Design review of the part built by this model. Coordinates are the model's own, in mm. Coordinates: 2 decimals unless noted, no trailing zeros. Loops run counter-clockwise (first coordinate to the right, second up) from the corner with the lowest first, then second, coordinate; pieces in that order, holes last. Notation, with made-up numbers: (6, 13) -> (32, 13) arc R7 cw to (32, 24) -> close; hole circle Ø5 at (-12, 32.25). An arc over 180 degrees is marked (long way). Use CSV: the item, a comma, the result in double quotes.
```python
from build123d import *

# Parameters (mm, degrees)
SKETCH1_R           = 1.6
SKETCH1_R_2         = 1.65
SKETCH1_R_3         = 1.5
BOSS_EXTRUDE1_DEPTH = 4
FILLET1_R           = 4
FILLET2_R           = 10


with BuildPart() as part:
    # Sketch1 → Boss-Extrude1 (new body)
    with BuildSketch(Plane.XY):
        with BuildLine():
            Line((0, 0), (96, 0))
            Line((96, 0), (96, 20))
            Line((96, 20), (80, 31.52))
            Line((80, 31.52), (80, 126))
            Line((80, 126), (16, 126))
            Line((16, 126), (16, 70.5))
            Line((16, 70.5), (36.610950109, 67.962533624))
            ThreePointArc((36.610950109, 67.962533624), (41, 63), (36.610950109, 58.037466376))
            Line((36.610950109, 58.037466376), (16, 55.5))
            Line((16, 55.5), (16, 31.52))
            Line((16, 31.52), (0, 20))
            Line((0, 20), (0, 0))
        make_face()
        with Locations((4.15, 5)):
            Circle(SKETCH1_R, mode=Mode.SUBTRACT)
        with Locations((12.65, 5)):
            Circle(SKETCH1_R, mode=Mode.SUBTRACT)
        with Locations((12.65, 15)):
            Circle(SKETCH1_R, mode=Mode.SUBTRACT)
        with Locations((4.15, 15)):
            Circle(SKETCH1_R, mode=Mode.SUBTRACT)
        with Locations(Location((91.85, 5, 0), (0, 0, 180))):
            Circle(SKETCH1_R, mode=Mode.SUBTRACT)
        with Locations(Location((83.35, 5, 0), (0, 0, 180))):
            Circle(SKETCH1_R, mode=Mode.SUBTRACT)
        with Locations(Location((83.35, 15, 0), (0, 0, 180))):
            Circle(SKETCH1_R, mode=Mode.SUBTRACT)
        with Locations(Location((91.85, 15, 0), (0, 0, 180))):
            Circle(SKETCH1_R, mode=Mode.SUBTRACT)
        with Locations((48, 3)):
            Circle(SKETCH1_R, mode=Mode.SUBTRACT)
        with Locations((23.5, 123)):
            Circle(SKETCH1_R, mode=Mode.SUBTRACT)
        with Locations((72.5, 123)):
            Circle(SKETCH1_R, mode=Mode.SUBTRACT)
        with Locations((64, 71)):
            Circle(SKETCH1_R_2, mode=Mode.SUBTRACT)
        with Locations((64, 55)):
            Circle(SKETCH1_R_2, mode=Mode.SUBTRACT)
        with Locations((46, 63)):
            Circle(SKETCH1_R_3, mode=Mode.SUBTRACT)
        with BuildLine():
            Line((45.35, 122.6), (45.35, 109.4))
            ThreePointArc((45.35, 109.4), (43.75, 107.8), (42.15, 109.4))
            Line((42.15, 109.4), (42.15, 122.6))
            ThreePointArc((42.15, 122.6), (43.75, 124.2), (45.35, 122.6))
        make_face(mode=Mode.SUBTRACT)
        with BuildLine():
            Line((50.65, 109.4), (50.65, 122.6))
            ThreePointArc((50.65, 122.6), (52.25, 124.2), (53.85, 122.6))
            Line((53.85, 122.6), (53.85, 109.4))
            ThreePointArc((53.85, 109.4), (52.25, 107.8), (50.65, 109.4))
        make_face(mode=Mode.SUBTRACT)
    extrude(amount=BOSS_EXTRUDE1_DEPTH)

    # Fillet1
    fillet1_edges = [part.edges().sort_by_distance(p)[0] for p in [
        (16, 55.5, 2),
        (16, 70.5, 2),
        (16, 126, 2),
        (80, 126, 2),
        (96, 0, 2),
        (0, 0, 2),
    ]]
    fillet(fillet1_edges, radius=FILLET1_R)

    # Fillet2
    fillet2_edges = [part.edges().sort_by_distance(p)[0] for p in [
        (0, 20, 2),
        (16, 31.52, 2),
        (80, 31.52, 2),
        (96, 20, 2),
    ]]
    fillet(fillet2_edges, radius=FILLET2_R)


solid = part.part
```
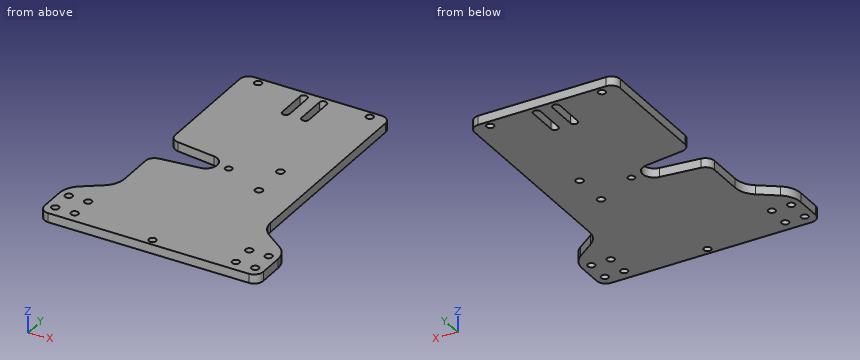
Item 1: Add section C-C (x = 64). Give the boundary of the cut face in (y, z), then the cut area to 3 significant figures.
Checked values:
outline,"(0, 0) -> (53.35, 0) -> (53.35, 4) -> (0, 4) -> close; (56.65, 0) -> (69.35, 0) -> (69.35, 4) -> (56.65, 4) -> close; (72.65, 0) -> (126, 0) -> (126, 4) -> (72.65, 4) -> close"
area,"478 mm^2"
Item 2: Add section A-A (y = 63). Give the boundary of the cut face in (x, z), then the cut area to 3 significant figures.
Checked values:
outline,"(41, 0) -> (44.5, 0) -> (44.5, 4) -> (41, 4) -> close; (47.5, 0) -> (80, 0) -> (80, 4) -> (47.5, 4) -> close"
area,"144 mm^2"
Item 3: Add section D-D (z = 2.7). State how many separate pieces and enclosed holes the cut face has, then the cut area to 3 significant figures.
Checked values:
separate pieces,"1"
enclosed holes,"16"
area,"8,370 mm^2"
Item 4: To check wall thickness, follow line 1 along Y through (x, z) = (91.85, 2.45); line 2 along Y through (x, z) = (64, 1.9); line 3 along Y through (x, z) = (72.5, 1.95). State the ranges of each line that lie inside material, in increasing order.
Checked values:
line 1,"0 to 3.4, 6.6 to 13.4, 16.6 to 22.99"
line 2,"0 to 53.35, 56.65 to 69.35, 72.65 to 126"
line 3,"0 to 121.4, 124.6 to 126"
Item 5: Clearance check with flat-ended pins moving along their axes: pin 1 (3.5 mm diameter, centred on x = 23.5, y = 123, fed in from -Z); pin 2 (1.5 mm diameter, centred on y = 90.5, z = 2, fed in from +X); pin 3 (2 mm diameter, centred on y = 108, z = 1, fed in from -X). State where each tip first meets the part, or that it passes through.
Checked values:
pin 1,"z = 0"
pin 2,"x = 80"
pin 3,"x = 16"
Item 6: Add section B-B (x = 52.25). Give the boundary of the cut face in (y, z).
Checked values:
outline,"(0, 0) -> (107.8, 0) -> (107.8, 4) -> (0, 4) -> close; (124.2, 0) -> (126, 0) -> (126, 4) -> (124.2, 4) -> close"
